Work out the finished part from the listing and answer in its coordinate system (mm). A direction names the side the tool comes from. Give positions to 0.01 mm unless a question says otherwise; leave off trailing zeros. Write each loop counter-clockwise with the first axis right and the second up, starting at its lowest first coordinate (ties: lowest second). Pieces come first, ordered by that corner, then holes. Notation, with made-up numbers: (0.5, -1.5) - (33.5, -1.5) arc R34 cw to (33.5, 37.5) - close; hole circle Ø1 at (-5, 30.25). An arc over 180 degrees is marked (long way). Write item = value, one per line.
from build123d import *

# Parameters (mm, degrees)
SKETCH_5_R      = 3
EXTRUDE_1_DEPTH = 50
SKETCH_6_R      = 3
EXTRUDE_2_DEPTH = 50
SKETCH_7_R      = 3
EXTRUDE_3_DEPTH = 50


with BuildPart() as part:
    # 草图4 → 旋转10 (revolve)
    with BuildSketch(Plane.XY):
        with BuildLine():
            Line((0, -7.5), (0, 7.5))
            ThreePointArc((0, 7.5), (-7.5, 0), (0, -7.5))
        make_face()
    revolve(axis=Axis((0, -7.5, 0), (0, 1, 0)))

    # 草图5 → 凸台-拉伸1 (add)
    with BuildSketch(Plane(origin=(0, 0, 0), x_dir=(1, 0, 0), z_dir=(0, 1, 0))):
        with Locations(Location((0, 0, 0), (0, 0, 90))):
            Circle(SKETCH_5_R)
    extrude(amount=EXTRUDE_1_DEPTH)

    # 草图6 → 凸台-拉伸2 (add)
    with BuildSketch(Plane.XY):
        with Locations(Location((0, 0, 0), (0, 0, 180))):
            Circle(SKETCH_6_R)
    extrude(amount=EXTRUDE_2_DEPTH)

    # 草图7 → 凸台-拉伸3 (add)
    with BuildSketch(Plane(origin=(0, 0, 0), x_dir=(0, 0, -1), z_dir=(1, 0, 0))):
        with Locations(Location((0, 0, 0), (0, 0, 180))):
            Circle(SKETCH_7_R)
    extrude(amount=EXTRUDE_3_DEPTH)


solid = part.part
1. Straight lines are drawn through the part: line 1 (X direction, y = -2.5, z = 2); line 2 (Y direction, x = 19, z = -2.5); line 3 (X direction, y = 21, z = 1). For each, find the intervals that lie inside material, in ascending order.
Solution:
line_1 = -6.78 to 6.78
line_2 = -1.66 to 1.66
line_3 = -2.83 to 2.83
2. A tool of negligible diameter and unlimited length cuts with its end or side. For faces 1 (the cylindrical face through (28.14, -0.9, 2.86)), 2 (the cylindrical face through (-0.9, 28.14, -2.86)), 3 (the flat face through (0, 50, 0)), 4 (the cylindrical face through (-2.86, -0.9, 28.14)), 5 (the flat face through (50, 0, 0)), from which of +Z, -Z, +X, -X, +Y, -Y can it reach the whole face along a straight path? Write none if from no direction.
Solution:
face_1 = +X
face_2 = +Y
face_3 = +Z, -Z, +X, -X, +Y
face_4 = +Z
face_5 = +Z, -Z, +X, +Y, -Y
3. Find section C-C, the plane x = 28. Give the vertices of the cut face in (y, z).
Solution:
outline = circle Ø6 at (0, 0)
4. Find section A-A, the plane y = 0. Give the vertices of the cut face in (x, z), then the cut area to 3 significant figures.
Solution:
outline = (-3, 6.87) arc R7.5 ccw (long way) to (6.87, -3) - (50, -3) - (50, 3) - (6.87, 3) arc R7.5 ccw to (3, 6.87) - (3, 50) - (-3, 50) - close
area = 689 mm^2
5. Given pin 1 (4 mm diameter, centred on x = -0.5, y = 38.5, fed in from -Z), flat-ended and moving along its own axis, determine where the tip first touches the part or whether it passes through.
Solution:
pin_1 = -3
